Here's how the part is built. I have some questions about the finished solid (model axes, mm). Give positions to 0.01 mm unless a question says otherwise; leave off trailing zeros. Write each loop counter-clockwise with the first axis right and the second up, starting at its lowest first coordinate (ties: lowest second). Pieces come first, ordered by that corner, then holes. Notation, with made-up numbers: (54.5, -0.75) - (67.5, -0.75) arc R20 ccw to (67.5, 31.25) - close; hole circle Ø8 at (-15.5, 57). An arc over 180 degrees is marked (long way). Use a Markdown table: item, result.
```python
from build123d import *

# Parameters (mm, degrees)
BOSS_EXTRUDE1_DEPTH                        = 3
CUT_EXTRUDE1_REACH                         = 178.78
SKETCH2_R                                  = 2.1
SKETCH2_W                                  = 44.07
SKETCH2_H                                  = 66
MIRROR4_AT_THE_SECOND_PLANE_COPY_1_REACH   = 178.78
MIRROR4_AT_THE_SECOND_PLANE_COPY_1_SKETC_R = 2.1
MIRROR4_AT_THE_SECOND_PLANE_COPY_1_SKETC_W = 44.07
MIRROR4_AT_THE_SECOND_PLANE_COPY_1_SKETC_H = 66
SKETCH3_R                                  = 2.1
CUT_EXTRUDE2_DEPTH                         = 177.780230795
CUT_EXTRUDE5_REACH                         = 178.78
SKETCH6_R                                  = 1.35
SKETCH6_R_2                                = 2.1
SKETCH6_R_3                                = 1.3
CUT_EXTRUDE12_REACH                        = 178.78
SKETCH13_R                                 = 1.5
MIRROR6_AT_THE_SECOND_PLANE_COPY_1_REACH   = 178.78
MIRROR6_AT_THE_SECOND_PLANE_COPY_1_SKETC_R = 1.5


with BuildPart() as part:
    # Sketch1 → Boss-Extrude1 (new body)
    with BuildSketch(Plane(origin=(0, 0, 0), x_dir=(1, 0, 0), z_dir=(0, 1, 0))):
        with BuildLine():
            Line((-117.293435451, 93.5), (117.293435451, 93.5))
            ThreePointArc((117.293435451, 93.5), (150, 0), (117.293435451, -93.5))
            Line((117.293435451, -93.5), (-117.293435451, -93.5))
            ThreePointArc((-117.293435451, -93.5), (-150, 0), (-117.293435451, 93.5))
        make_face()
    extrude(amount=BOSS_EXTRUDE1_DEPTH)

    # Sketch2 → Cut-Extrude1 (cut, up to next)
    with BuildSketch(Plane(origin=(0, 3, 0), x_dir=(1, 0, 0), z_dir=(0, 1, 0)), mode=Mode.PRIVATE) as cut_extrude1_sk1:
        with Locations(Location((-109.548435451, 50.5, 0), (0, 0, 270))):
            Circle(SKETCH2_R)
    cut_extrude1_tool1 = extrude(cut_extrude1_sk1.sketch, amount=-CUT_EXTRUDE1_REACH, mode=Mode.PRIVATE) & part.part
    # Sketch2 → Cut-Extrude1 (cut, up to next)
    with BuildSketch(Plane(origin=(0, 3, 0), x_dir=(1, 0, 0), z_dir=(0, 1, 0)), mode=Mode.PRIVATE) as cut_extrude1_sk2:
        with Locations(Location((-50.968435451, 50.5, 0), (0, 0, 270))):
            Circle(SKETCH2_R)
    cut_extrude1_tool2 = extrude(cut_extrude1_sk2.sketch, amount=-CUT_EXTRUDE1_REACH, mode=Mode.PRIVATE) & part.part
    # Sketch2 → Cut-Extrude1 (cut, up to next)
    with BuildSketch(Plane(origin=(0, 3, 0), x_dir=(1, 0, 0), z_dir=(0, 1, 0)), mode=Mode.PRIVATE) as cut_extrude1_sk3:
        with Locations((-80.258435451, 60.5)):
            Rectangle(SKETCH2_W, SKETCH2_H)
    cut_extrude1_tool3 = extrude(cut_extrude1_sk3.sketch, amount=-CUT_EXTRUDE1_REACH, mode=Mode.PRIVATE) & part.part
    cut_extrude1_1 = cut_extrude1_tool1.solids().sort_by_distance((-109.548435, 3, -50.5))[0]
    add(cut_extrude1_1, mode=Mode.SUBTRACT)
    cut_extrude1_2 = cut_extrude1_tool2.solids().sort_by_distance((-50.968435, 3, -50.5))[0]
    add(cut_extrude1_2, mode=Mode.SUBTRACT)
    cut_extrude1_3 = cut_extrude1_tool3.solids().sort_by_distance((-80.258435, 3, -60.5))[0]
    add(cut_extrude1_3, mode=Mode.SUBTRACT)
    cut_extrude1 = cut_extrude1_1 + cut_extrude1_2 + cut_extrude1_3  # Cut-Extrude1 as one shape, for the pattern or mirror that repeats it

    # Mirror4: Cut-Extrude1 across plane
    add(cut_extrude1.mirror(Plane.XY), mode=Mode.SUBTRACT)

    # Mirror4 at the second plane: Cut-Extrude1 across plane
    add(cut_extrude1.mirror(Plane(origin=(0, 0, 0), x_dir=(0, 0, 1), z_dir=(1, 0, 0))), mode=Mode.SUBTRACT)

    # Mirror4 at the second plane copy 1 sketc → Mirror4 at the second plane copy 1 (cut, up to next)
    with BuildSketch(Plane(origin=(0, 3, 0), x_dir=(-1, 0, 0), z_dir=(0, 1, 0)), mode=Mode.PRIVATE) as mirror4_at_the_second_plane_copy_1_sk1:
        with Locations(Location((-109.548435451, 50.5, 0), (0, 0, 270))):
            Circle(MIRROR4_AT_THE_SECOND_PLANE_COPY_1_SKETC_R)
    mirror4_at_the_second_plane_copy_1_tool1 = extrude(mirror4_at_the_second_plane_copy_1_sk1.sketch, amount=-MIRROR4_AT_THE_SECOND_PLANE_COPY_1_REACH, mode=Mode.PRIVATE) & part.part
    # Mirror4 at the second plane copy 1 sketc → Mirror4 at the second plane copy 1 (cut, up to next)
    with BuildSketch(Plane(origin=(0, 3, 0), x_dir=(-1, 0, 0), z_dir=(0, 1, 0)), mode=Mode.PRIVATE) as mirror4_at_the_second_plane_copy_1_sk2:
        with Locations(Location((-50.968435451, 50.5, 0), (0, 0, 270))):
            Circle(MIRROR4_AT_THE_SECOND_PLANE_COPY_1_SKETC_R)
    mirror4_at_the_second_plane_copy_1_tool2 = extrude(mirror4_at_the_second_plane_copy_1_sk2.sketch, amount=-MIRROR4_AT_THE_SECOND_PLANE_COPY_1_REACH, mode=Mode.PRIVATE) & part.part
    # Mirror4 at the second plane copy 1 sketc → Mirror4 at the second plane copy 1 (cut, up to next)
    with BuildSketch(Plane(origin=(0, 3, 0), x_dir=(-1, 0, 0), z_dir=(0, 1, 0)), mode=Mode.PRIVATE) as mirror4_at_the_second_plane_copy_1_sk3:
        with Locations((-80.258435451, 60.5)):
            Rectangle(MIRROR4_AT_THE_SECOND_PLANE_COPY_1_SKETC_W, MIRROR4_AT_THE_SECOND_PLANE_COPY_1_SKETC_H)
    mirror4_at_the_second_plane_copy_1_tool3 = extrude(mirror4_at_the_second_plane_copy_1_sk3.sketch, amount=-MIRROR4_AT_THE_SECOND_PLANE_COPY_1_REACH, mode=Mode.PRIVATE) & part.part
    add(mirror4_at_the_second_plane_copy_1_tool1.solids().sort_by_distance((109.548435, 3, 50.5))[0], mode=Mode.SUBTRACT)
    add(mirror4_at_the_second_plane_copy_1_tool2.solids().sort_by_distance((50.968435, 3, 50.5))[0], mode=Mode.SUBTRACT)
    add(mirror4_at_the_second_plane_copy_1_tool3.solids().sort_by_distance((80.258435, 3, 60.5))[0], mode=Mode.SUBTRACT)

    # Sketch3 → Cut-Extrude2 (cut, through all)
    with BuildSketch(Plane(origin=(0, 3, 0), x_dir=(1, 0, 0), z_dir=(0, 1, 0))):
        with Locations(Location((-42.993435451, 82.5, 0), (0, 0, 270))):
            Circle(SKETCH3_R)
        with Locations(Location((42.993435451, 82.5, 0), (0, 0, 270))):
            Circle(SKETCH3_R)
        with Locations(Location((-113.813435451, 76, 0), (0, 0, 270))):
            Circle(SKETCH3_R)
        with Locations(Location((130.463435451, 47.48, 0), (0, 0, 270))):
            Circle(SKETCH3_R)
        with Locations(Location((130.463435451, -47.48, 0), (0, 0, 90))):
            Circle(SKETCH3_R)
        with Locations(Location((42.993435451, -82.5, 0), (0, 0, 90))):
            Circle(SKETCH3_R)
        with Locations(Location((-42.993435451, -82.5, 0), (0, 0, 90))):
            Circle(SKETCH3_R)
        with Locations(Location((-113.813435451, -76, 0), (0, 0, 90))):
            Circle(SKETCH3_R)
    extrude(amount=-CUT_EXTRUDE2_DEPTH, mode=Mode.SUBTRACT)

    # Sketch6 → Cut-Extrude5 (cut, up to next)
    with BuildSketch(Plane(origin=(0, 3, 0), x_dir=(1, 0, 0), z_dir=(0, 1, 0)), mode=Mode.PRIVATE) as cut_extrude5_sk1:
        with Locations(Location((-31.526564549, -31, 0), (0, 0, 270))):
            Circle(SKETCH6_R)
    cut_extrude5_tool1 = extrude(cut_extrude5_sk1.sketch, amount=-CUT_EXTRUDE5_REACH, mode=Mode.PRIVATE) & part.part
    # Sketch6 → Cut-Extrude5 (cut, up to next)
    with BuildSketch(Plane(origin=(0, 3, 0), x_dir=(1, 0, 0), z_dir=(0, 1, 0)), mode=Mode.PRIVATE) as cut_extrude5_sk2:
        with Locations(Location((17.473435451, -31, 0), (0, 0, 270))):
            Circle(SKETCH6_R)
    cut_extrude5_tool2 = extrude(cut_extrude5_sk2.sketch, amount=-CUT_EXTRUDE5_REACH, mode=Mode.PRIVATE) & part.part
    # Sketch6 → Cut-Extrude5 (cut, up to next)
    with BuildSketch(Plane(origin=(0, 3, 0), x_dir=(1, 0, 0), z_dir=(0, 1, 0)), mode=Mode.PRIVATE) as cut_extrude5_sk3:
        with Locations(Location((114.153435451, 37.485, 0), (0, 0, 270))):
            Circle(SKETCH6_R_2)
    cut_extrude5_tool3 = extrude(cut_extrude5_sk3.sketch, amount=-CUT_EXTRUDE5_REACH, mode=Mode.PRIVATE) & part.part
    # Sketch6 → Cut-Extrude5 (cut, up to next)
    with BuildSketch(Plane(origin=(0, 3, 0), x_dir=(1, 0, 0), z_dir=(0, 1, 0)), mode=Mode.PRIVATE) as cut_extrude5_sk4:
        with Locations(Location((114.153435451, -37.485, 0), (0, 0, 270))):
            Circle(SKETCH6_R_2)
    cut_extrude5_tool4 = extrude(cut_extrude5_sk4.sketch, amount=-CUT_EXTRUDE5_REACH, mode=Mode.PRIVATE) & part.part
    # Sketch6 → Cut-Extrude5 (cut, up to next)
    with BuildSketch(Plane(origin=(0, 3, 0), x_dir=(1, 0, 0), z_dir=(0, 1, 0)), mode=Mode.PRIVATE) as cut_extrude5_sk5:
        with Locations(Location((46.363435451, 37.485, 0), (0, 0, 270))):
            Circle(SKETCH6_R_2)
    cut_extrude5_tool5 = extrude(cut_extrude5_sk5.sketch, amount=-CUT_EXTRUDE5_REACH, mode=Mode.PRIVATE) & part.part
    # Sketch6 → Cut-Extrude5 (cut, up to next)
    with BuildSketch(Plane(origin=(0, 3, 0), x_dir=(1, 0, 0), z_dir=(0, 1, 0)), mode=Mode.PRIVATE) as cut_extrude5_sk6:
        with Locations(Location((-24.5, -35, 0), (0, 0, 270))):
            Circle(SKETCH6_R_3)
    cut_extrude5_tool6 = extrude(cut_extrude5_sk6.sketch, amount=-CUT_EXTRUDE5_REACH, mode=Mode.PRIVATE) & part.part
    # Sketch6 → Cut-Extrude5 (cut, up to next)
    with BuildSketch(Plane(origin=(0, 3, 0), x_dir=(1, 0, 0), z_dir=(0, 1, 0)), mode=Mode.PRIVATE) as cut_extrude5_sk7:
        with Locations(Location((24.5, -35, 0), (0, 0, 270))):
            Circle(SKETCH6_R_3)
    cut_extrude5_tool7 = extrude(cut_extrude5_sk7.sketch, amount=-CUT_EXTRUDE5_REACH, mode=Mode.PRIVATE) & part.part
    # Sketch6 → Cut-Extrude5 (cut, up to next)
    with BuildSketch(Plane(origin=(0, 3, 0), x_dir=(1, 0, 0), z_dir=(0, 1, 0)), mode=Mode.PRIVATE) as cut_extrude5_sk8:
        with Locations(Location((30.463435451, -29.615, 0), (0, 0, 270))):
            Circle(SKETCH6_R_2)
    cut_extrude5_tool8 = extrude(cut_extrude5_sk8.sketch, amount=-CUT_EXTRUDE5_REACH, mode=Mode.PRIVATE) & part.part
    add(cut_extrude5_tool1.solids().sort_by_distance((-31.526565, 3, 31))[0], mode=Mode.SUBTRACT)
    add(cut_extrude5_tool2.solids().sort_by_distance((17.473435, 3, 31))[0], mode=Mode.SUBTRACT)
    add(cut_extrude5_tool3.solids().sort_by_distance((114.153435, 3, -37.485))[0], mode=Mode.SUBTRACT)
    add(cut_extrude5_tool4.solids().sort_by_distance((114.153435, 3, 37.485))[0], mode=Mode.SUBTRACT)
    add(cut_extrude5_tool5.solids().sort_by_distance((46.363435, 3, -37.485))[0], mode=Mode.SUBTRACT)
    add(cut_extrude5_tool6.solids().sort_by_distance((-24.5, 3, 35))[0], mode=Mode.SUBTRACT)
    add(cut_extrude5_tool7.solids().sort_by_distance((24.5, 3, 35))[0], mode=Mode.SUBTRACT)
    add(cut_extrude5_tool8.solids().sort_by_distance((30.463435, 3, 29.615))[0], mode=Mode.SUBTRACT)

    # Sketch13 → Cut-Extrude12 (cut, up to next)
    with BuildSketch(Plane(origin=(0, 3, 0), x_dir=(1, 0, 0), z_dir=(0, 1, 0)), mode=Mode.PRIVATE) as cut_extrude12_sk1:
        with Locations((-102.293435451, 27.5)):
            Circle(SKETCH13_R)
    cut_extrude12_tool1 = extrude(cut_extrude12_sk1.sketch, amount=-CUT_EXTRUDE12_REACH, mode=Mode.PRIVATE) & part.part
    # Sketch13 → Cut-Extrude12 (cut, up to next)
    with BuildSketch(Plane(origin=(0, 3, 0), x_dir=(1, 0, 0), z_dir=(0, 1, 0)), mode=Mode.PRIVATE) as cut_extrude12_sk2:
        with Locations((-58.223435451, 27.5)):
            Circle(SKETCH13_R)
    cut_extrude12_tool2 = extrude(cut_extrude12_sk2.sketch, amount=-CUT_EXTRUDE12_REACH, mode=Mode.PRIVATE) & part.part
    cut_extrude12_1 = cut_extrude12_tool1.solids().sort_by_distance((-102.293435, 3, -27.5))[0]
    add(cut_extrude12_1, mode=Mode.SUBTRACT)
    cut_extrude12_2 = cut_extrude12_tool2.solids().sort_by_distance((-58.223435, 3, -27.5))[0]
    add(cut_extrude12_2, mode=Mode.SUBTRACT)
    cut_extrude12 = cut_extrude12_1 + cut_extrude12_2  # Cut-Extrude12 as one shape, for the pattern or mirror that repeats it

    # Mirror6: Cut-Extrude12 across plane
    add(cut_extrude12.mirror(Plane(origin=(0, 0, 0), x_dir=(0, 0, 1), z_dir=(1, 0, 0))), mode=Mode.SUBTRACT)

    # Mirror6 at the second plane: Cut-Extrude12 across plane
    add(cut_extrude12.mirror(Plane.XY), mode=Mode.SUBTRACT)

    # Mirror6 at the second plane copy 1 sketc → Mirror6 at the second plane copy 1 (cut, up to next)
    with BuildSketch(Plane(origin=(0, 3, 0), x_dir=(-1, 0, 0), z_dir=(0, 1, 0)), mode=Mode.PRIVATE) as mirror6_at_the_second_plane_copy_1_sk1:
        with Locations((-102.293435451, 27.5)):
            Circle(MIRROR6_AT_THE_SECOND_PLANE_COPY_1_SKETC_R)
    mirror6_at_the_second_plane_copy_1_tool1 = extrude(mirror6_at_the_second_plane_copy_1_sk1.sketch, amount=-MIRROR6_AT_THE_SECOND_PLANE_COPY_1_REACH, mode=Mode.PRIVATE) & part.part
    # Mirror6 at the second plane copy 1 sketc → Mirror6 at the second plane copy 1 (cut, up to next)
    with BuildSketch(Plane(origin=(0, 3, 0), x_dir=(-1, 0, 0), z_dir=(0, 1, 0)), mode=Mode.PRIVATE) as mirror6_at_the_second_plane_copy_1_sk2:
        with Locations((-58.223435451, 27.5)):
            Circle(MIRROR6_AT_THE_SECOND_PLANE_COPY_1_SKETC_R)
    mirror6_at_the_second_plane_copy_1_tool2 = extrude(mirror6_at_the_second_plane_copy_1_sk2.sketch, amount=-MIRROR6_AT_THE_SECOND_PLANE_COPY_1_REACH, mode=Mode.PRIVATE) & part.part
    add(mirror6_at_the_second_plane_copy_1_tool1.solids().sort_by_distance((102.293435, 3, 27.5))[0], mode=Mode.SUBTRACT)
    add(mirror6_at_the_second_plane_copy_1_tool2.solids().sort_by_distance((58.223435, 3, 27.5))[0], mode=Mode.SUBTRACT)


solid = part.part
```
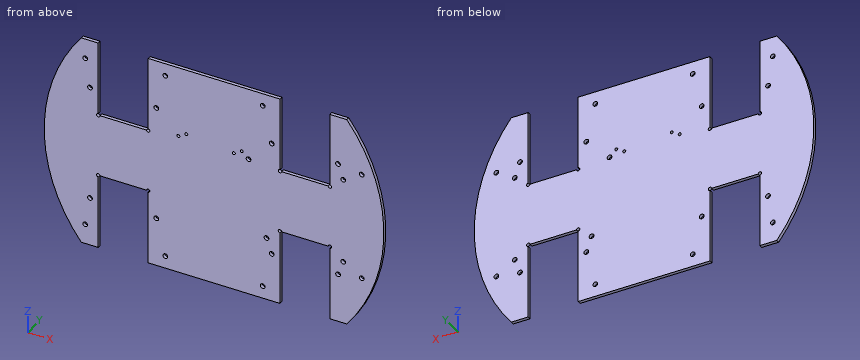
Item 1: If we section it at A-A, the plane x = 94.5: Write out the boundary of the cut face in (y, z), plus the area to 3 significant figures.
Values:
| item | result |
|---|---|
| outline | (0, -27.5) - (3, -27.5) - (3, 27.5) - (0, 27.5) - close |
| area | 165 mm2 |
Item 2: If we section it at B-B, the plane y = 1.4: Count the separate pieces of the cut face and the enclosed holes in it, plus the area to 3 significant figures.
Values:
| item | result |
|---|---|
| separate pieces | 1 |
| enclosed holes | 24 |
| area | 40,200 mm2 |
Item 3: Will these pins go through, and if not, where does the flat tip stop? pin 1 Ø1.5 at (y, z) = (2, 47) entering from +X; pin 2 Ø3.5 at (x, z) = (114.15, -37.48) entering from -Y; pin 3 Ø0.9 at (y, z) = (2, 55) entering from -X; pin 4 Ø1 at (x, y) = (-91, 0.5) entering from +Z.
Values:
| item | result |
|---|---|
| pin 1 | stops at x = 142.69 |
| pin 2 | passes through |
| pin 3 | stops at x = -139.73 |
| pin 4 | stops at z = 27.5 |
Item 4: I need wall thicknesses on line 1 along Z through (x, y) = (-113.5, 0.9); line 2 along Z through (x, y) = (41.5, 0.8); line 3 along X through (y, z) = (2.8, -63.5). Which ranges of each line are inside material? Lowest first, please. Write a range as [from, to].
Values:
| item | result |
|---|---|
| line 1 | z = [-93.5, -78.08], [-73.92, 73.92], [78.08, 93.5] |
| line 2 | z = [-93.5, -83.98], [-81.02, 81.02], [83.98, 93.5] |
| line 3 | x = [-135.9, -102.29], [-58.22, 58.22], [102.29, 135.9] |
